from build123d import *

# Parameters (mm, degrees)
ESBO_O1_R                = 3.97
RESSALTO_EXTRUS_O1_DEPTH = 22.5
ESBO_O2_W                = 36.5
ESBO_O2_H                = 9.5
CORTE_EXTRUS_O1_DEPTH    = 25
CHANFRO1_SIZE            = 7


with BuildPart() as part:
    # Esboço1 → Ressalto-extrusão1 (new body, symmetric)
    with BuildSketch(Plane.XY):
        Polygon((30, -12.5), (-30, -12.5), (-30, 12.5), (-19.930804426, 24.5), (30.977490779, 24.5), (50.977490779, 24.5), (50.977490779, 12.5), align=None)
        with Locations((-20, 0)):
            Circle(ESBO_O1_R, mode=Mode.SUBTRACT)
        with Locations((20, 0)):
            Circle(ESBO_O1_R, mode=Mode.SUBTRACT)
    extrude(amount=RESSALTO_EXTRUS_O1_DEPTH, both=True)

    # Esboço2 → Corte-extrusão1 (cut)
    with BuildSketch(Plane(origin=(50.977490779, 0, 0), x_dir=(0, 0, -1), z_dir=(1, 0, 0))):
        with Locations((0, 18.5)):
            Rectangle(ESBO_O2_W, ESBO_O2_H)
    extrude(amount=-CORTE_EXTRUS_O1_DEPTH, mode=Mode.SUBTRACT)

    # Chanfro1
    chanfro1_edges = [part.edges().sort_by_distance(p)[0] for p in [
        (-30, -12.5, 0),
    ]]
    chamfer(chanfro1_edges, length=CHANFRO1_SIZE)


solid = part.part
Source: CAD feature listing. Evaluate the final solid. Frame: model axes, mm. A direction names the side the tool comes from. Give positions to 0.01 mm unless a question says otherwise; leave off trailing zeros. Write each loop counter-clockwise with the first axis right and the second up, starting at its lowest first coordinate (ties: lowest second). Pieces come first, ordered by that corner, then holes. Notation, with made-up numbers: M -39,61.5 L -12,61.5 A15 cw -12,74.5 Z; hole C 83.25,42 d5. An arc over 180 degrees is marked long. Return JSON: item names as keys, results as strings. Group by question number.
1) Cut plane C-C, the plane y = -3. Output: boundary loops of the cut face in (x, z).
2) Cut plane D-D, the plane x = 34. Output: boundary loops of the cut face in (y, z), plus the area to 3 significant figures.
3) Cut plane A-A, the plane x = 20. Output: boundary loops of the cut face in (y, z).
4) Pull-direction query (Y, two-part tool) for faces 1 (the face through (16, 24.5, 0)), 2 (the face through (4, -12.5, 0)), 3 (the face through (-22.93, 2.68, -0.32)), 4 (the face through (50.977, 24, 0)); classes: pulls with the +Y half, pulls with the -Y half, needs draft (parallel to the pull), parting line crosses it, or undercut.
5) Material intervals for line 1 along Y through (x, z) = (20, -12); line 2 along Z through (x, y) = (36.5, 18); line 3 along X through (y, z) = (3.5, -6), sorted ascending. Write a range as [from, to].
6) Set-up query: faces 5 (the face through (-25.036, 18.416, 0.315)), 6 (the face through (39, 18, 18.25)). Return all of +Z, -Z, +X, -X, +Y, -Y with unobstructed straight access to the full face (end or side cutting, diameter ignored); none if empty.
7) Cut plane B-B, the plane z = 2. Output: boundary loops of the cut face in (x, y).
8) Pin query (flat end, axial travel): P1, Ø5, axis at x = -20, y = 0, coming from the +Z side; P2, Ø3, axis at y = 18.5, z = -5, coming from the +X side; P3, Ø1, axis at x = 32, z = -5.5, coming from the -Y side. Return the tip coordinate at first contact, or that it passes through.
Recorded:
{
 "1": {"outline": "M -30,-22.5 L -22.6,-22.5 L -22.6,22.5 L -30,22.5 Z; M -17.4,-22.5 L 17.4,-22.5 L 17.4,22.5 L -17.4,22.5 Z; M 22.6,-22.5 L 37.97,-22.5 L 37.97,22.5 L 22.6,22.5 Z"},
 "2": {"outline": "M -7.73,-22.5 L 24.5,-22.5 L 24.5,22.5 L -7.73,22.5 Z; hole M 13.75,-18.25 L 23.25,-18.25 L 23.25,18.25 L 13.75,18.25 Z", "area": "1,100 mm²"},
 "3": {"outline": "M -12.5,-22.5 L -3.97,-22.5 L -3.97,22.5 L -12.5,22.5 Z; M 3.97,-22.5 L 24.5,-22.5 L 24.5,22.5 L 3.97,22.5 Z"},
 "4": {"face 1": "pulls with the +Y half", "face 2": "pulls with the -Y half", "face 3": "undercut", "face 4": "needs draft"},
 "5": {"line 1": "y = [-12.5, -3.97], [3.97, 24.5]", "line 2": "z = [-22.5, -18.25], [18.25, 22.5]", "line 3": "x = [-30, -21.87], [-18.13, 18.13], [21.87, 43.43]"},
 "6": {"face 5": "+Z, -Z, -X, +Y", "face 6": "+X"},
 "7": {"outline": "M -30,-5.5 L -23,-12.5 L 30,-12.5 L 50.98,12.5 L 50.98,13.75 L 25.98,13.75 L 25.98,23.25 L 50.98,23.25 L 50.98,24.5 L -19.93,24.5 L -30,12.5 Z; hole C -20,0 d7.94; hole C 20,0 d7.94"},
 "8": {"P1": "passes through", "P2": "stops at x = 25.98", "P3": "stops at y = -10.71"}
}
